Check sheet for the modelled part. Datum: model origin and axes. Units: mm. Round coordinates to 2 decimals unless told otherwise and drop trailing zeros. Write each loop counter-clockwise with the first axis right and the second up, starting at its lowest first coordinate (ties: lowest second). Pieces come first, ordered by that corner, then holes.
Item 1: Go/stop test with a flat-tipped pin: pin 1 Ø5.5 at (y, z) = (300, -940) entering from -X. Record where the tip stops, or that it passes through.
Item 2: Cross-section at A-A on y = -135.5. Enter the section's corners in (x, z).
Item 3: Material ranges on line 1 (Y direction, x = 0.7, z = -305); line 2 (Y direction, x = 0.8, z = -940); line 3 (Z direction, x = 1.5, y = -260), recorded low to high.
Item 4: Cross-section at B-B on x = 0.95. Count the separate pieces of the cut face and the enclosed holes in it, plus the area to 3 significant figures.
Item 5: Cross-section at C-C on z = 14. Enter the section's corners in (x, y).
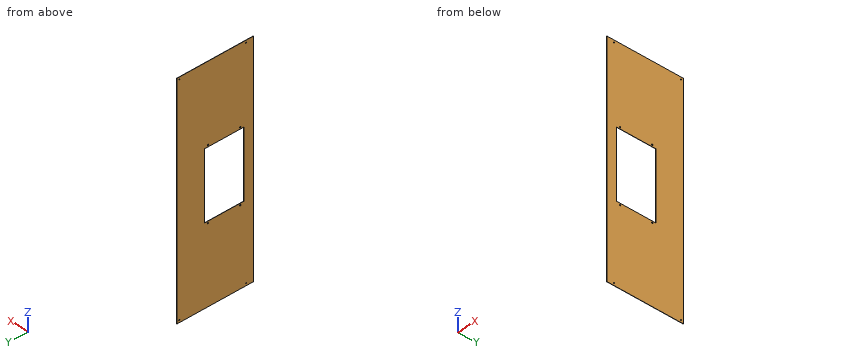
from build123d import *

# Parameters (mm, degrees)
SKETCH1_W   = 1920
SKETCH1_H   = 640
SKETCH1_R   = 4.5
SKETCH1_R_2 = 5.5
SKETCH1_W_2 = 580
SKETCH1_H_2 = 330
THICKEN1_T1 = 2


with BuildPart() as body_1:
    # Sketch1 → Surface-Plane1: a flat surface bounded by the sketch
    with BuildSketch(Plane(origin=(0, 0, 0), x_dir=(0, 0, -1), z_dir=(1, 0, 0)), mode=Mode.PRIVATE) as surface_plane1_1_region:
        Rectangle(SKETCH1_W, SKETCH1_H)
        with Locations((-940, 300)):
            Circle(SKETCH1_R, mode=Mode.SUBTRACT)
        with Locations((940, 300)):
            Circle(SKETCH1_R, mode=Mode.SUBTRACT)
        with Locations((940, -260)):
            Circle(SKETCH1_R, mode=Mode.SUBTRACT)
        with Locations((-940, -260)):
            Circle(SKETCH1_R, mode=Mode.SUBTRACT)
        with Locations((-305, 60)):
            Circle(SKETCH1_R_2, mode=Mode.SUBTRACT)
        with Locations((305, 60)):
            Circle(SKETCH1_R_2, mode=Mode.SUBTRACT)
        with Locations((305, -210)):
            Circle(SKETCH1_R_2, mode=Mode.SUBTRACT)
        with Locations((-305, -210)):
            Circle(SKETCH1_R_2, mode=Mode.SUBTRACT)
        with Locations((0, -75)):
            Rectangle(SKETCH1_W_2, SKETCH1_H_2, mode=Mode.SUBTRACT)
    surface_plane1_1 = surface_plane1_1_region.sketch.faces()[0]
    add(Solid.thicken(surface_plane1_1, THICKEN1_T1))


solid = body_1.part
Response values:
1. pin 1: passes through
2. outline: (0, -960) - (2, -960) - (2, -290) - (0, -290) - close; (0, 290) - (2, 290) - (2, 960) - (0, 960) - close
3. line 1: y = -320 to -215.5, -204.5 to 54.5, 65.5 to 320
3. line 2: y = -320 to -264.5, -255.5 to 295.5, 304.5 to 320
3. line 3: z = -960 to -944.5, -935.5 to 935.5, 944.5 to 960
4. separate pieces: 1
4. enclosed holes: 9
4. area: 1,040,000 mm2
5. outline: (0, -320) - (2, -320) - (2, -240) - (0, -240) - close; (0, 90) - (2, 90) - (2, 320) - (0, 320) - close
